For this review, take the finished solid that the model builds, in its own axes (mm). Face numbers are marked on the shaded views. Round coordinates to 2 decimals unless told otherwise and drop trailing zeros. Order: outer loops, then holes, each group sorted by start corner. A loop starts at its lowest first (then second) coordinate and runs counter-clockwise, first axis right, second up. Notation, with made-up numbers: M -29,10.25 L -23,10.25 A21 cw -23,34.25 Z; hole C 89.25,43 d6. An arc over 180 degrees is marked long. Answer in a Markdown table with one row per item. Add a question column.
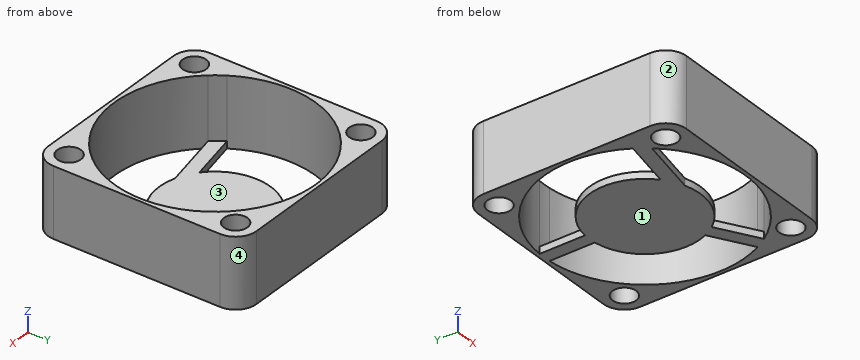
```python
from build123d import *
from build123d.topology import SkipClean

# Parameters (mm, degrees)
BOSS_EXTRU_1_DEPTH      = 10
ENL_V_MAT_EXTRU_1_DEPTH = 9
D_GAGEMENT_M32_D        = 3.4


with BuildPart() as part:
    # Esquisse1 → Boss.-Extru.1 (new body)
    with BuildSketch(Plane.XY.offset(6.5)):
        with BuildLine():
            Line((-12, -15), (12, -15))
            ThreePointArc((12, -15), (14.121320344, -14.121320344), (15, -12))
            Line((15, -12), (15, 12))
            ThreePointArc((15, 12), (14.121320344, 14.121320344), (12, 15))
            Line((12, 15), (-12, 15))
            ThreePointArc((-12, 15), (-14.121320344, 14.121320344), (-15, 12))
            Line((-15, 12), (-15, -12))
            ThreePointArc((-15, -12), (-14.121320344, -14.121320344), (-12, -15))
        make_face()
        with BuildLine():
            Line((6.409501891, -4.787304619), (12.033174962, -8.090284317))
            ThreePointArc((12.033174962, -8.090284317), (0.780346659, -14.478986812), (-11.093944394, -9.336723075))
            Line((-11.093944394, -9.336723075), (-2.459433312, -7.612567752))
            ThreePointArc((-2.459433312, -7.612567752), (2.428227417, -7.622579066), (6.409501891, -4.787304619))
        make_face(mode=Mode.SUBTRACT)
        with BuildLine():
            Line((12.979808931, -6.463324231), (7.350678361, -3.157139153))
            ThreePointArc((7.350678361, -3.157139153), (6.92820323, 4), (0.941176471, 7.944443772))
            Line((0.941176471, 7.944443772), (0.941176471, 14.469422478))
            ThreePointArc((0.941176471, 14.469422478), (12.56954374, 7.228870601), (12.979808931, -6.463324231))
        make_face(mode=Mode.SUBTRACT)
        with BuildLine():
            Line((-5.143653135, -6.127220612), (-12.367309381, -7.569653802))
            ThreePointArc((-12.367309381, -7.569653802), (-12.874431786, 6.670757541), (-0.948221665, 14.468962495))
            Line((-0.948221665, 14.468962495), (-0.948221665, 7.943605962))
            ThreePointArc((-0.948221665, 7.943605962), (-7.666470815, 2.285875158), (-5.143653135, -6.127220612))
        make_face(mode=Mode.SUBTRACT)
    extrude(amount=-BOSS_EXTRU_1_DEPTH)

    # Esquisse2 → Enlèv. mat.-Extru.1 (cut)
    with SkipClean():  # the faces are left unmerged after this step: merging them gives an invalid solid
        with BuildSketch(Plane.XY.offset(6.5)):
            with BuildLine():
                Line((-11.093944394, -9.336723075), (-2.459433312, -7.612567752))
                ThreePointArc((-2.459433312, -7.612567752), (2.428227417, -7.622579066), (6.409501891, -4.787304619))
                Line((6.409501891, -4.787304619), (12.033174962, -8.090284317))
                ThreePointArc((12.033174962, -8.090284317), (12.532920274, -7.292181389), (12.979808931, -6.463324231))
                Line((12.979808931, -6.463324231), (7.350678361, -3.157139153))
                ThreePointArc((7.350678361, -3.157139153), (6.92820323, 4), (0.941176471, 7.944443772))
                Line((0.941176471, 7.944443772), (0.941176471, 14.469422478))
                ThreePointArc((0.941176471, 14.469422478), (-0.003530097, 14.49999957), (-0.948221665, 14.468962495))
                Line((-0.948221665, 14.468962495), (-0.948221665, 7.943605962))
                ThreePointArc((-0.948221665, 7.943605962), (-7.666470815, 2.285875158), (-5.143653135, -6.127220612))
                Line((-5.143653135, -6.127220612), (-12.367309381, -7.569653802))
                ThreePointArc((-12.367309381, -7.569653802), (-11.763853137, -8.477131553), (-11.093944394, -9.336723075))
            make_face()
        extrude(amount=-ENL_V_MAT_EXTRU_1_DEPTH, mode=Mode.SUBTRACT)

    # Dégagement M32 (through all)
    with Locations(Plane.XY.offset(6.5)):
        with Locations((-12, 12), (-12, -12), (12, -12), (12, 12)):
            Hole(D_GAGEMENT_M32_D / 2)


solid = part.part
```
1. The part is to be moulded in two halves that separate along Y. For the marked faces 1, 2, 3 and 4, say which applies: pulls with the +Y half, pulls with the -Y half, needs draft (parallel to the pull), parting line crosses it, or undercut.
2. Clearance check with a flat-ended pin moving along its axis: pin 1 Ø2 at (x, y) = (12, 12) entering from -Z. State where the tip first meets the part, or that it passes through.
3. Consider section C-C on x = -9. Write out the cut boundary in (y, z).
4. To check wall thickness, follow probe 1 along X at (y, z) = (0, 5.75); probe 2 along X at (y, z) = (-11, 6.25); probe 3 along X at (y, z) = (10.75, 0.5). State the ranges of each line that lie inside material, in increasing order. Write a range as [from, to].
5. Consider section A-A on z = 0.25. Write out the cut boundary in (x, y).
6. Consider section B-B on y = 4. Write out the cut boundary in (x, z), plus the area to 3 significant figures.
Solved:
| question | item | result |
|---|---|---|
| 1 | face 1 | needs draft |
| 1 | face 2 | pulls with the -Y half |
| 1 | face 3 | undercut |
| 1 | face 4 | pulls with the +Y half |
| 2 | pin 1 | passes through |
| 3 | outline | M -15,-3.5 L -11.37,-3.5 L -11.37,6.5 L -15,6.5 Z; M -8.92,-3.5 L -6.9,-3.5 L -6.9,-2.5 L -8.92,-2.5 Z; M 11.37,-3.5 L 15,-3.5 L 15,6.5 L 11.37,6.5 Z |
| 4 | probe 1 | x = [-15, -14.5], [14.5, 15] |
| 4 | probe 2 | x = [-15, -13.37], [-10.63, -9.45], [9.45, 10.63], [13.37, 15] |
| 4 | probe 3 | x = [-15, -13.15], [-10.85, -9.73], [9.73, 10.85], [13.15, 15] |
| 5 | outline | M -15,-12 A3 ccw -12,-15 L 12,-15 A3 ccw 15,-12 L 15,12 A3 ccw 12,15 L -12,15 A3 ccw -15,12 Z; hole C 0,0 d29; hole C -12,-12 d3.4; hole C -12,12 d3.4; hole C 12,-12 d3.4; hole C 12,12 d3.4 |
| 6 | outline | M -15,-3.5 L -13.94,-3.5 L -13.94,6.5 L -15,6.5 Z; M -6.93,-3.5 L 6.93,-3.5 L 6.93,-2.5 L -6.93,-2.5 Z; M 13.94,-3.5 L 15,-3.5 L 15,6.5 L 13.94,6.5 Z |
| 6 | area | 35.1 mm^2 |
